Input: part model. Units: mm. Frame: model coordinates. A direction names the side the tool comes from. Coordinates: 2 decimals unless noted, no trailing zeros. Order: outer loops, then holes, each group sorted by start corner. A loop starts at its lowest first (then second) coordinate and runs counter-clockwise, first axis right, second up. Notation, with made-up numbers: (-7, -7.5) -> (15, -7.5) arc R18 ccw to (15, 19.5) -> close; hole circle Ø5 at (15.5, 3.5). An arc over 180 degrees is marked (long way). One line per item, written item: value. Start each with the question number.
from build123d import *

# Parameters (mm, degrees)
SKETCH1_R           = 7.4
BOSS_EXTRUDE1_DEPTH = 5
SKETCH2_R           = 4.9
BOSS_EXTRUDE2_DEPTH = 10
SKETCH13_OUTSIDE_W  = 21.95
SKETCH13_OUTSIDE_H  = 21.95
SKETCH13_OUTSIDE_R  = 4
CUT_EXTRUDE4_DEPTH  = 5.5
THREAD2_PITCH       = 1.25
SKETCH5_W           = 3
SKETCH5_H           = 14.8
CUT_EXTRUDE5_DEPTH  = 2.5


with BuildPart() as part:
    # Sketch1 → Boss-Extrude1 (new body)
    with BuildSketch(Plane(origin=(0, 0, 0), x_dir=(1, 0, 0), z_dir=(0, 1, 0))):
        with Locations(Location((0, 0, 0), (0, 0, 270))):
            Circle(SKETCH1_R)
    extrude(amount=BOSS_EXTRUDE1_DEPTH)

    # Sketch2 → Boss-Extrude2 (add)
    with BuildSketch(Plane(origin=(0, 5, 0), x_dir=(1, 0, 0), z_dir=(0, 1, 0))):
        with Locations(Location((0, 0, 0), (0, 0, 270))):
            Circle(SKETCH2_R)
    extrude(amount=BOSS_EXTRUDE2_DEPTH)

    # Sketch13 outside → Cut-Extrude4 (cut)
    with BuildSketch(Plane(origin=(0, 15, 0), x_dir=(1, 0, 0), z_dir=(0, 1, 0))):
        Rectangle(SKETCH13_OUTSIDE_W, SKETCH13_OUTSIDE_H)
        with Locations(Location((0, 0, 0), (0, 0, 270))):
            Circle(SKETCH13_OUTSIDE_R, mode=Mode.SUBTRACT)
    extrude(amount=-CUT_EXTRUDE4_DEPTH, mode=Mode.SUBTRACT)

    # Thread2: the profile of Thread Profile4 profile screwed along a right-hand helix of 4.4 turns, 8 arcs to a turn; built about Z, then put on its axis
    thread2_z = Axis((0, 0, 0), (0, 0, 1))
    thread2_corners = [(3.9997, 0, -0.000173205), (4.676582344, 0, 0.390624998), (4.676582344, 0, 0.546874998), (3.9997, 0, 0.937673202)]
    with BuildLine(mode=Mode.PRIVATE) as thread2_profile:
        Line(thread2_corners[0], thread2_corners[1])
        Line(thread2_corners[1], thread2_corners[2])
        Line(thread2_corners[2], thread2_corners[3])
        Line(thread2_corners[3], thread2_corners[0])
    thread2_cap = Face(thread2_profile.wire())
    thread2_turn_angles = [0, 22.5, 45, 67.5, 90, 112.5, 135, 157.5, 180, 202.5, 225, 247.5, 270, 292.5, 315, 337.5, 360]
    thread2_turn_weights = [1, 0.9238795325112867, 1, 0.9238795325112867, 1, 0.9238795325112867, 1, 0.9238795325112867, 1, 0.9238795325112867, 1, 0.9238795325112867, 1, 0.9238795325112867, 1, 0.9238795325112867, 1]
    thread2_turn_rails = [Edge.make_bspline([Vector(p[0], p[1], 0).rotate(thread2_z, thread2_turn_angles[k]) / thread2_turn_weights[k] + Vector(0, 0, p[2] + THREAD2_PITCH * thread2_turn_angles[k] / 360) for k in range(17)], [0, 0, 0, 1, 1, 2, 2, 3, 3, 4, 4, 5, 5, 6, 6, 7, 7, 8, 8, 8], 2, thread2_turn_weights) for p in thread2_corners]
    thread2_turn_sides = [Face.make_surface_from_curves(thread2_turn_rails[p[0]], thread2_turn_rails[p[1]]) for p in [(0, 1), (1, 2), (2, 3), (3, 0)]]
    thread2_last_angles = [1440, 1462.5, 1485, 1507.5, 1530, 1552.5, 1575, 1579.5, 1584]
    thread2_last_weights = [1, 0.9238795325112867, 1, 0.9238795325112867, 1, 0.9238795325112867, 1, 0.996917333733128, 1]
    thread2_last_rails = [Edge.make_bspline([Vector(p[0], p[1], 0).rotate(thread2_z, thread2_last_angles[k]) / thread2_last_weights[k] + Vector(0, 0, p[2] + THREAD2_PITCH * thread2_last_angles[k] / 360) for k in range(9)], [0, 0, 0, 1, 1, 2, 2, 3, 3, 4, 4, 4], 2, thread2_last_weights) for p in thread2_corners]
    thread2_last_sides = [Face.make_surface_from_curves(thread2_last_rails[p[0]], thread2_last_rails[p[1]]) for p in [(0, 1), (1, 2), (2, 3), (3, 0)]]
    thread2 = Plane(origin=(0, 15, 0), x_dir=(-1, 0, 0), z_dir=(0, -1, 0)) * Solid(Shell([*[p.moved(Location((0, 0, THREAD2_PITCH * i))) for i in range(4) for p in thread2_turn_sides], *thread2_last_sides, thread2_cap, thread2_cap.rotate(thread2_z, 1584).moved(Location((0, 0, THREAD2_PITCH * 1584 / 360)))]))
    add(thread2)

    # Sketch5 → Cut-Extrude5 (cut)
    with BuildSketch(Plane.XZ):
        Rectangle(SKETCH5_W, SKETCH5_H)
    extrude(amount=-CUT_EXTRUDE5_DEPTH, mode=Mode.SUBTRACT)


solid = part.part
1) Section query A-A, the plane y = 7.25. Return the cut outline in (x, z).
2) Mould query, pull axis X, two halves, no side actions, for faces 1 (the cylindrical face through (-2.834, 2.465, 6.836)), 2 (the flat face through (-1.5, 1, 0)), 3 (the flat face through (4, 0, 0)). Classes: +X half, -X half, draft (parallel to the pull), parting line (faces both ways), or undercut.
3) Pin query (flat end, axial travel): pin 1 Ø5 at (x, y) = (-3, 12) entering from +Z; pin 2 Ø1.5 at (y, z) = (10.5, 4.5) entering from +X; pin 3 Ø0.8 at (y, z) = (2, 1.5) entering from +X; pin 4 Ø3 at (x, y) = (1, 4) entering from +Z. Return the tip coordinate at first contact, or that it passes through.
4) Access query for faces 4 (the flat face through (-5, 5, 2)), 5 (the flat face through (4, 9.5, -2)), 6 (the flat face through (0, 2.5, 0)). Directions: +Z, -Z, +X, -X, +Y, -Y. A direction counts if a zero-diameter tool reaches every point of the face in a straight line with its end or side. Return the directions, or none.
5) Ray query, line 1 along Y through (x, z) = (-4.25, 1.25); line 2 along Y through (x, z) = (-3.5, -3); line 3 along Y through (x, z) = (5, -0.5). Return the intervals inside material, ascending. Write a range as from..to.
Entries:
1. outline: circle Ø9.8 at (0, 0)
2. face 1: parting line
2. face 2: undercut
2. face 3: draft
3. pin 1: stops at z = 4.65
3. pin 2: stops at x = 2.57
3. pin 3: stops at x = 7.32
3. pin 4: stops at z = 7.4
4. face 4: +Y
4. face 5: none
4. face 6: +Z, -Z, -Y
5. line 1: y = 0..9.81, 10.62..11.06, 11.87..12.31, 13.12..13.56
5. line 2: y = 0..9.51, 10.52..10.76, 11.77..12.01, 13.02..13.26, 14.27..14.51
5. line 3: y = 0..5
